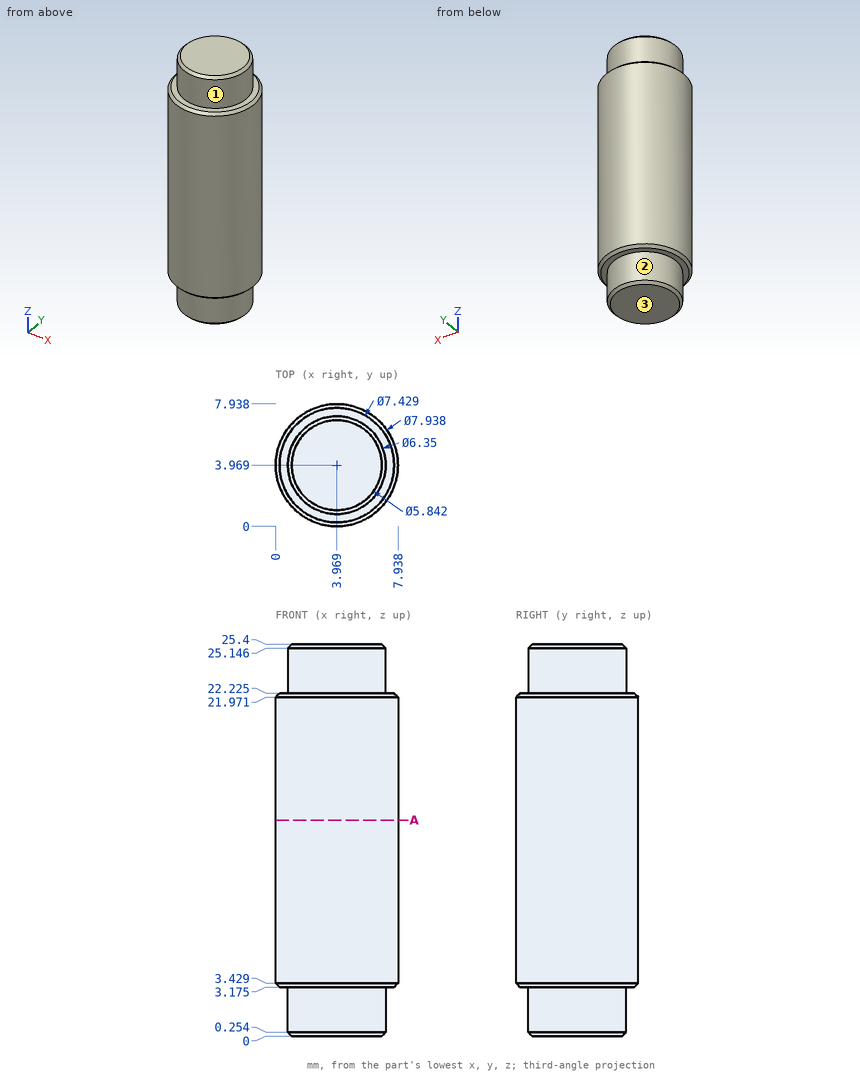
Could you check a few things on this drawing? It's one solid part, dimensions in mm from its lowest x, y, z. A direction names the side the tool comes from. Round coordinates to 2 decimals unless told otherwise and drop trailing zeros. Order: outer loops, then holes, each group sorted by start corner. A loop starts at its lowest first (then second) coordinate and runs counter-clockwise, first axis right, second up.
Q1. Which directions (+Z, -Z, +X, -X, +Y, -Y) give clear straight access to the entire face, cutting with the end or side of a thin tool? Please do the marked faces 1, 2 and 3.
Geometry says:
face 1: +Z
face 2: -Z
face 3: -Z, +X, -X, +Y, -Y
Q2. Please list where these lines run through material, in increasing order: probe 1 along Z at (x, y) = (2, 6.5) (1 decimal); probe 2 along X at (y, z) = (2, 23); probe 3 along X at (y, z) = (2.75, 7.5) (1 decimal).
Geometry says:
probe 1: z = 3.2 to 22.2
probe 2: x = 1.48 to 6.46
probe 3: x = 0.2 to 7.7
Q3. I'm going to push a flat-ended pin straight in: P1, Ø4, axis at x = 1, z = 3, coming from the -Y side. Where does the tip first touch, or does it pass through?
Geometry says:
P1: stops at y = 0.13
Q4. Imagine slicing it at A-A, the plane z = 14. List the corners of the cut face in (x, y) for me.
Geometry says:
outline: circle Ø7.94 at (3.97, 3.97)
